Read the model definition and answer for the solid it produces. Units are mm, in the model's axes. A direction names the side the tool comes from. Round coordinates to 2 decimals unless told otherwise and drop trailing zeros. Write each loop counter-clockwise with the first axis right and the second up, starting at its lowest first coordinate (ties: lowest second). Pieces come first, ordered by that corner, then holes.
from build123d import *

# Parameters (mm, degrees)
RESSALTO_EXTRUS_O1_DEPTH = 25
ESPELHAR1_START          = -25
ESPELHAR1_DEPTH          = 50
ESBO_O10_R               = 3
CORTE_EXTRUS_O6_DEPTH    = 44.5
RESSALTO_EXTRUS_O2_START = 0.75
RESSALTO_EXTRUS_O2_DEPTH = 9
ESBO_O12_R               = 2.5
CORTE_EXTRUS_O7_DEPTH    = 189.180392443
PADR_O_LINEAR1_COUNT     = 13
PADR_O_LINEAR1_PITCH     = 10
CORTE_EXTRUS_O8_DEPTH    = 189.180392443
FILETE1_R                = 5


# Read off the part's stored shape, not the designer's step: Espelhar1
with BuildPart() as part:
    # Esboço2 → Ressalto-extrusão1 (new, symmetric)
    with BuildSketch(Plane(origin=(0, 0, 0), x_dir=(0, 0, -1), z_dir=(1, 0, 0))):
        with BuildLine():
            Line((14.172351725, -19.333068153), (9.75, -45.76))
            Line((9.75, -45.76), (0.75, -45.76))
            Line((0.75, -45.76), (0.75, -15.982412208))
            ThreePointArc((0.75, -15.982412208), (15.995602448, 0.375103096), (0, 16))
            Line((0, 16), (0, 20.76))
            ThreePointArc((0, 20.76), (18.307093974, 9.789173112), (17.265058969, -11.528024063))
            ThreePointArc((17.265058969, -11.528024063), (15.304550089, -15.266439288), (14.172351725, -19.333068153))
        make_face()
    extrude(amount=RESSALTO_EXTRUS_O1_DEPTH, both=True)

    # Espelhar1 outline → Espelhar1 (add)
    with BuildSketch(Plane.YZ.offset(ESPELHAR1_START)):
        with BuildLine():
            Line((-19.333068153, 14.172351725), (-45.76, 9.75))
            Line((-45.76, 9.75), (-45.76, 0.75))
            Line((-45.76, 0.75), (-15.982412208, 0.75))
            ThreePointArc((-15.982412208, 0.75), (0.375103096, 15.995602448), (16, 0))
            Line((16, 0), (20.76, 0))
            ThreePointArc((20.76, 0), (9.789173112, 18.307093974), (-11.528024063, 17.265058969))
            ThreePointArc((-11.528024063, 17.265058969), (-15.266439288, 15.304550089), (-19.333068153, 14.172351725))
        make_face()
    extrude(amount=ESPELHAR1_DEPTH)

    # Esboço10 → Corte-extrusão6 (cut, symmetric)
    with BuildSketch(Plane.XY):
        with Locations(Location((-12.5, -37.76, 0), (0, 0, 90))):
            Circle(ESBO_O10_R)
        with Locations(Location((12.5, -37.76, 0), (0, 0, 90))):
            Circle(ESBO_O10_R)
    extrude(amount=CORTE_EXTRUS_O6_DEPTH, both=True, mode=Mode.SUBTRACT)

    # Esboço11 → Ressalto-extrusão2 (add)
    with BuildSketch(Plane.XY.offset(RESSALTO_EXTRUS_O2_START)):
        with BuildLine():
            Line((-25, -45.76), (25, -45.76))
            Line((25, -45.76), (25, -184))
            Line((25, -184), (13, -184))
            ThreePointArc((13, -184), (-14.37934254, -117.183349367), (-25, -45.76))
        make_face()
    extrude(amount=RESSALTO_EXTRUS_O2_DEPTH)

    # Esboço12 → Corte-extrusão7 (cut, through all)
    with BuildSketch(Plane.XY.offset(9.75)):
        with Locations((19, -178)):
            Circle(ESBO_O12_R)
    corte_extrus_o7 = extrude(amount=-CORTE_EXTRUS_O7_DEPTH, mode=Mode.SUBTRACT)

    # Padrão linear1: Corte-extrusão7 ×13
    with Locations(*[(0, i * PADR_O_LINEAR1_PITCH, 0) for i in range(1, PADR_O_LINEAR1_COUNT)]):
        add(corte_extrus_o7, mode=Mode.SUBTRACT)

    # Esboço13 → Corte-extrusão8 (cut, through all)
    with BuildSketch(Plane.XY.offset(9.75)):
        with BuildLine():
            Line((-16.219640416, -60), (12, -60))
            Line((12, -60), (12, -146))
            Line((12, -146), (3, -146))
            ThreePointArc((3, -146), (-10.033576546, -103.765155415), (-16.219640416, -60))
        make_face()
    extrude(amount=-CORTE_EXTRUS_O8_DEPTH, mode=Mode.SUBTRACT)

    # Filete1
    filete1_edges = [part.edges().sort_by_distance(p)[0] for p in [
        (13, -184, 5.25),
        (25, -184, 5.25),
    ]]
    fillet(filete1_edges, radius=FILETE1_R)


solid = part.part
Q1. Flat-ended cylindrical pins translate along their axes: pin 1 Ø6.5 at (x, y) = (19, -78) entering from -Z; pin 2 Ø2.5 at (y, z) = (-105, 6.5) entering from -X; pin 3 Ø4.5 at (x, z) = (-3, 4) entering from -Y. Find the tip coordinate at first contact, or state that the pin passes through.
Verdict:
pin 1: stops at z = 0.75
pin 2: stops at x = -17.74
pin 3: stops at y = -156.08
Q2. Section B-B (y = -98) is taken. Determine the outline of the cut face in (x, z), then the cut area to 3 significant figures.
Verdict:
outline: (-18.98, 0.75) - (-11.26, 0.75) - (-11.26, 9.75) - (-18.98, 9.75) - close; (12, 0.75) - (16.5, 0.75) - (16.5, 9.75) - (12, 9.75) - close; (21.5, 0.75) - (25, 0.75) - (25, 9.75) - (21.5, 9.75) - close
area: 141 mm2
Q3. Which of the six approach directions +Z, -Z, +X, -X, +Y, -Y give full straight-line access (tool end or side, diameter ignored) to faces 5 (the flat face through (0, -45.76, -5)), 6 (the flat face through (-2, -60, 5)), 7 (the cylindrical face through (-0.35, -15.211, 15.326))?
Verdict:
face 5: -Z, +X, -X, -Y
face 6: +Z, -Z
face 7: +Z, +X, -X, -Y
Q4. Determine the mould class of faces 1 (the flat face through (25, -64, 3)), 2 (the flat face through (17, -114, 9.75)), 3 (the cylindrical face through (17.16, -96.31, 5.31)), 4 (the cylindrical face through (-13.4, -34.9, 6.1)) for opening direction X: pulls with the +X half, pulls with the -X half, needs draft (parallel to the pull), parting line crosses it, or undercut.
Verdict:
face 1: pulls with the +X half
face 2: needs draft
face 3: undercut
face 4: undercut
Q5. Straight lines are drawn through the part: probe 1 along X at (y, z) = (-37.76, 9); probe 2 along Y at (x, z) = (-12.5, -6.5); probe 3 along Z at (x, y) = (-16.5, -60). For each, find the intervals that lie inside material, in ascending order.
Verdict:
probe 1: x = -25 to -15.5, -9.5 to 9.5, 15.5 to 25
probe 2: y = -45.76 to -40.76, -34.76 to -14.62, 14.62 to 19.72
probe 3: z = 0.75 to 9.75
Q6. Section C-C (x = 7) is taken. Determine the outline of the cut face in (y, z).
Verdict:
outline: (-172.7, 0.75) - (-146, 0.75) - (-146, 9.75) - (-172.7, 9.75) - close; (-60, 0.75) - (-15.98, 0.75) arc R16 cw (long way) to (-15.98, -0.75) - (-45.76, -0.75) - (-45.76, -9.75) - (-19.33, -14.17) arc R20 cw to (-11.53, -17.27) arc R20.76 ccw (long way) to (-11.53, 17.27) arc R20 cw to (-19.33, 14.17) - (-45.76, 9.75) - (-60, 9.75) - close
Q7. Section D-D (y = -31.5) is taken. Determine the outline of the cut face in (x, z).
Verdict:
outline: (-25, -12.14) - (25, -12.14) - (25, -0.75) - (-25, -0.75) - close; (-25, 0.75) - (25, 0.75) - (25, 12.14) - (-25, 12.14) - close
Q8. Section A-A (x = -12.5) is taken. Determine the outline of the cut face in (y, z).
Verdict:
outline: (-123.73, 0.75) - (-91.43, 0.75) - (-91.43, 9.75) - (-123.73, 9.75) - close; (-60, 0.75) - (-40.76, 0.75) - (-40.76, 10.59) - (-45.76, 9.75) - (-60, 9.75) - close; (-45.76, -9.75) - (-40.76, -10.59) - (-40.76, -0.75) - (-45.76, -0.75) - close; (-34.76, -11.59) - (-19.33, -14.17) arc R20 cw to (-11.53, -17.27) arc R20.76 ccw (long way) to (-11.53, 17.27) arc R20 cw to (-19.33, 14.17) - (-34.76, 11.59) - (-34.76, 0.75) - (-15.98, 0.75) arc R16 cw (long way) to (-15.98, -0.75) - (-34.76, -0.75) - close
